Part model, mm, in its own coordinate system. Face numbers are marked on the shaded views. Round coordinates to 2 decimals unless told otherwise and drop trailing zeros. Write each loop counter-clockwise with the first axis right and the second up, starting at its lowest first coordinate (ties: lowest second). Pieces come first, ordered by that corner, then holes. Notation, with made-up numbers: (-28.75, 70) -> (-5.75, 70) arc R18 cw to (-5.75, 100) -> close; hole circle Ø6 at (16.5, 64.25). An arc over 180 degrees is marked (long way). Return JSON: item names as keys, results as strings. Group by question number.
```python
from build123d import *

# Parameters (mm, degrees)
F0_R     = 44.95
F1_DEPTH = 130
F2_R     = 7.5
F2_R_2   = 5.5
F3_DEPTH = 10
F4_R     = 44.95
F4_R_2   = 26.5
F5_DEPTH = 30


with BuildPart() as f1:
    # F0 (on Top) → F1 (new body)
    with BuildSketch(Plane.XY):
        Circle(F0_R)
    extrude(amount=F1_DEPTH)

    # F2 (on face) → F3 (join)
    with BuildSketch(Plane.XY.offset(130)):
        Circle(F2_R)
        Circle(F2_R_2, mode=Mode.SUBTRACT)
        with Locations((-23, 0)):
            Circle(F2_R)
        with Locations((-23, 0)):
            Circle(F2_R_2, mode=Mode.SUBTRACT)
    extrude(amount=F3_DEPTH)

    # F4 (on face) → F5 (cut)
    with BuildSketch(Plane(origin=(0, 0, 0), x_dir=(1, 0, 0), z_dir=(0, 0, -1))):
        Circle(F4_R)
        Circle(F4_R_2, mode=Mode.SUBTRACT)
    extrude(amount=-F5_DEPTH, mode=Mode.SUBTRACT)


solid = f1.part
```
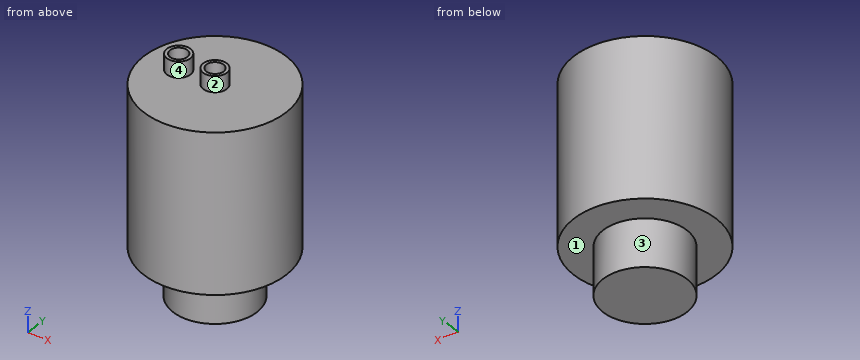
Item 1: Flat gauge pins, fed straight in: P1, Ø6, axis at x = -15, z = 58, coming from the -Y side; P2, Ø9, axis at x = 0, y = 0, coming from the +Z side; P3, Ø2, axis at x = -28.5, y = -5, coming from the -Z side. Where does each tip first touch, or does it go through?
Item 2: Wall check: L1, parallel to Y at x = 0, z = 136.25; L2, parallel to Z at x = -5, y = -2; L3, parallel to Z at x = -17, y = 32.5. Give the ranges that are in metal, low to high.
Item 3: Cut at D-D (x = -23). Write the cut outline in (y, z), then the cut area to 3 significant figures.
Item 4: Two-plate mould, pull along X, no slides. Class the marked faces 1, 2, 3 and 4: released by +X, released by -X, zero draft, split by the parting line, or undercut.
Item 5: Cut at A-A (y = 0). Write the cut outline in (x, z).
Item 6: Cut at C-C (z = 66). Write the cut outline in (x, y), then the cut area to 3 significant figures.
Item 7: Cut at B-B (x = 0). Write the cut outline in (y, z).
Checks:
{
 "1": {"P1": "stops at y = -43.32", "P2": "stops at z = 130", "P3": "stops at z = 30"},
 "2": {"L1": "y = -7.5 to -5.5, 5.5 to 7.5", "L2": "z = 0 to 130", "L3": "z = 30 to 130"},
 "3": {"outline": "(-38.62, 30) -> (-13.16, 30) -> (-13.16, 0) -> (13.16, 0) -> (13.16, 30) -> (38.62, 30) -> (38.62, 130) -> (7.5, 130) -> (7.5, 140) -> (5.5, 140) -> (5.5, 130) -> (-5.5, 130) -> (-5.5, 140) -> (-7.5, 140) -> (-7.5, 130) -> (-38.62, 130) -> close", "area": "8,550 mm2"},
 "4": {"face 1": "zero draft", "face 2": "undercut", "face 3": "split by the parting line", "face 4": "undercut"},
 "5": {"outline": "(-44.95, 30) -> (-26.5, 30) -> (-26.5, 0) -> (26.5, 0) -> (26.5, 30) -> (44.95, 30) -> (44.95, 130) -> (7.5, 130) -> (7.5, 140) -> (5.5, 140) -> (5.5, 130) -> (-5.5, 130) -> (-5.5, 140) -> (-7.5, 140) -> (-7.5, 130) -> (-15.5, 130) -> (-15.5, 140) -> (-17.5, 140) -> (-17.5, 130) -> (-28.5, 130) -> (-28.5, 140) -> (-30.5, 140) -> (-30.5, 130) -> (-44.95, 130) -> close"},
 "6": {"outline": "circle Ø89.9 at (0, 0)", "area": "6,350 mm2"},
 "7": {"outline": "(-44.95, 30) -> (-26.5, 30) -> (-26.5, 0) -> (26.5, 0) -> (26.5, 30) -> (44.95, 30) -> (44.95, 130) -> (7.5, 130) -> (7.5, 140) -> (5.5, 140) -> (5.5, 130) -> (-5.5, 130) -> (-5.5, 140) -> (-7.5, 140) -> (-7.5, 130) -> (-44.95, 130) -> close"}
}
